Read the model definition and answer for the solid it produces. Units are mm, in the model's axes. Coordinates: 2 decimals unless noted, no trailing zeros. Loops run counter-clockwise (first coordinate to the right, second up) from the corner with the lowest first, then second, coordinate; pieces in that order, holes last.
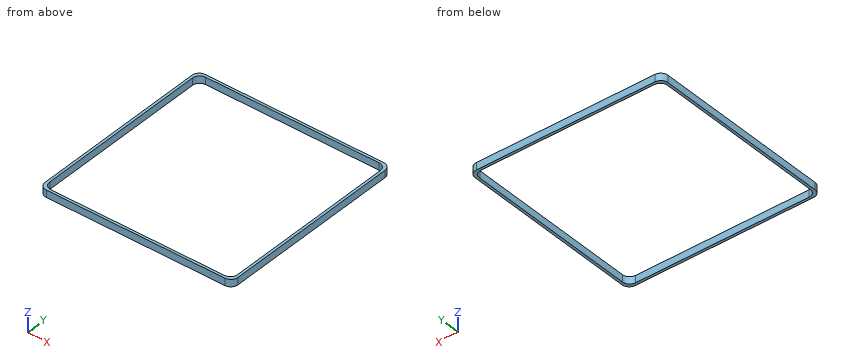
Autodesk Inventor part; units mm, degrees
ref_plane "YZ Plane" through (0, 0, 0) normal (1, 0, 0) x (0, 1, 0)
ref_plane "XZ Plane" through (0, 0, 0) normal (0, 1, 0) x (-1, 0, 0)
ref_plane "XY Plane" through (0, 0, 0) normal (0, 0, 1) x (1, 0, 0)
sketch "Sketch1" plane through (0, 0, 0) normal (0, 0, 1) x (1, 0, 0)
  line L0 (-875, -945) -> (875, -945)
  line L1 (945, -875) -> (945, 875)
  line L2 (875, 945) -> (-875, 945)
  line L3 (-945, 875) -> (-945, -875)
  line L4 (-945, -945) -> (945, 945) construction
  line L5 (945, -945) -> (-945, 945) construction
  line L6 (-850, -920) -> (850, -920)
  line L7 (920, -850) -> (920, 850)
  line L8 (850, 920) -> (-850, 920)
  line L9 (-920, 850) -> (-920, -850)
  line L10 (-920, -920) -> (920, 920) construction
  line L11 (920, -920) -> (-920, 920) construction
  arc A0 (-850, 920) -> (-920, 850) centre (-850, 850) ccw
  arc A1 (-875, 945) -> (-945, 875) centre (-875, 875) ccw
  arc A2 (920, 850) -> (850, 920) centre (850, 850) ccw
  arc A3 (945, 875) -> (875, 945) centre (875, 875) ccw
  arc A4 (850, -920) -> (920, -850) centre (850, -850) ccw
  arc A5 (875, -945) -> (945, -875) centre (875, -875) ccw
  arc A6 (-920, -850) -> (-850, -920) centre (-850, -850) ccw
  arc A7 (-945, -875) -> (-875, -945) centre (-875, -875) ccw
  point P0 (0, 0)
  dimension "d0" = 1890
  dimension "d1" = 1890
  dimension "d2" = 1840
  dimension "d3" = 1840
  dimension "d6" = 70
extrude "Extrusion1" add sketch "Sketch1" along normal blind 70
properties part number "Coil1or2"
Item 1: A cutting plane is placed at A-A on x = -586.5. Determine the outline of the cut face in (y, z), then the cut area to 3 significant figures.
Numbers:
outline: (-945, 0) - (-920, 0) - (-920, 70) - (-945, 70) - close; (920, 0) - (945, 0) - (945, 70) - (920, 70) - close
area: 3,500 mm2
Item 2: Find the intervals of material crossed by line 1 along Y through (x, z) = (-576.5, 62.5); line 2 along Y through (x, z) = (857, 62), in increasing order.
Numbers:
line 1: y = -945 to -920, 920 to 945
line 2: y = -945 to -919.65, 919.65 to 945
Item 3: A cutting plane is placed at C-C on z = 42. Determine the outline of the cut face in (x, y).
Numbers:
outline: (-945, -875) arc R70 ccw to (-875, -945) - (875, -945) arc R70 ccw to (945, -875) - (945, 875) arc R70 ccw to (875, 945) - (-875, 945) arc R70 ccw to (-945, 875) - close; hole (-920, -850) arc R70 ccw to (-850, -920) - (850, -920) arc R70 ccw to (920, -850) - (920, 850) arc R70 ccw to (850, 920) - (-850, 920) arc R70 ccw to (-920, 850) - close
